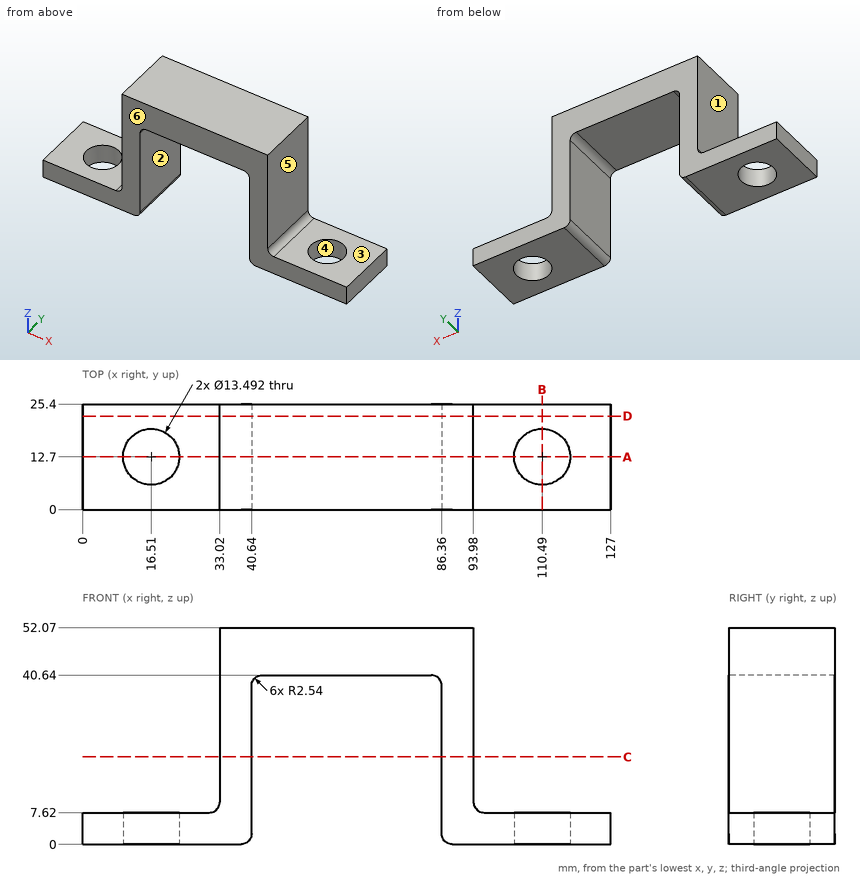
Answer from the drawing. Dimensions are ordinates in mm from the lowest x, y and z of the part. A direction names the side the tool comes from. Coordinates: 2 decimals unless noted, no trailing zeros. Write each loop counter-clockwise with the first axis right and the second up, starting at its lowest first coordinate (ties: lowest second). Pieces come first, ordered by that corner, then holes. Notation, with made-up numbers: (-1.75, 29) - (21.25, 29) arc R16 ccw to (21.25, 50) - close; hole circle Ø5 at (0, 77.5). An arc over 180 degrees is marked (long way). Return JSON: item names as keys, results as strings. Group by question number.
Q1. The part is cut by section B-B on x = 110.49. Write down the section's boundary in (y, z).
Q2. For a pull along X with two mould halves and no side action, classify the marked faces 4, 5 and 6 as +X half, -X half, draft (parallel to the pull), parting line (faces both ways), or undercut.
Q3. Which of the six approach directions +Z, -Z, +X, -X, +Y, -Y give full straight-line access (tool end or side, diameter ignored) to the marked faces 1, 2 and 3?
Q4. The part is cut by section A-A on y = 12.7. Write down the section's boundary in (x, z).
Q5. Find the intervals of material crossed by line 1 along X through (y, z) = (10.75, 25); line 2 along X through (y, z) = (11, 4.5); line 3 along Z through (x, y) = (97, 7), in increasing order. Write a range as [from, to].
Q6. The part is cut by section C-C on z = 21. Write down the section's boundary in (x, y), and give its area (3 significant figures).
Q7. The part is cut by section D-D on y = 22.5. Write down the section's boundary in (x, z), and give its area (3 significant figures).
Q8. Flat-ended cylindrical pins translate along their axes: pin 1 Ø7.5 at (x, y) = (60.5, 10.5) entering from -Z; pin 2 Ø12.5 at (y, z) = (15, 17) entering from -X; pin 3 Ø12.5 at (x, y) = (8, 10.5) entering from +Z. Find the tip coordinate at first contact, or state that the pin passes through.
Evaluation:
{
 "1": {"outline": "(0, 0) - (5.95, 0) - (5.95, 7.62) - (0, 7.62) - close; (19.45, 0) - (25.4, 0) - (25.4, 7.62) - (19.45, 7.62) - close"},
 "2": {"face 4": "undercut", "face 5": "+X half", "face 6": "draft"},
 "3": {"face 1": "+Z, -X, +Y, -Y", "face 2": "-Z, +Y, -Y", "face 3": "+Z, +X, +Y, -Y"},
 "4": {"outline": "(0, 0) - (9.76, 0) - (9.76, 7.62) - (0, 7.62) - close; (23.26, 0) - (38.1, 0) arc R2.54 ccw to (40.64, 2.54) - (40.64, 38.1) arc R2.54 cw to (43.18, 40.64) - (83.82, 40.64) arc R2.54 cw to (86.36, 38.1) - (86.36, 2.54) arc R2.54 ccw to (88.9, 0) - (103.74, 0) - (103.74, 7.62) - (96.52, 7.62) arc R2.54 cw to (93.98, 10.16) - (93.98, 52.07) - (33.02, 52.07) - (33.02, 10.16) arc R2.54 cw to (30.48, 7.62) - (23.26, 7.62) - close; (117.24, 0) - (127, 0) - (127, 7.62) - (117.24, 7.62) - close"},
 "5": {"line 1": "x = [33.02, 40.64], [86.36, 93.98]", "line 2": "x = [0, 9.98], [23.04, 40.64], [86.36, 103.96], [117.02, 127]", "line 3": "z = [0, 7.62]"},
 "6": {"outline": "(33.02, 0) - (40.64, 0) - (40.64, 25.4) - (33.02, 25.4) - close; (86.36, 0) - (93.98, 0) - (93.98, 25.4) - (86.36, 25.4) - close", "area": "387 mm2"},
 "7": {"outline": "(0, 0) - (38.1, 0) arc R2.54 ccw to (40.64, 2.54) - (40.64, 38.1) arc R2.54 cw to (43.18, 40.64) - (83.82, 40.64) arc R2.54 cw to (86.36, 38.1) - (86.36, 2.54) arc R2.54 ccw to (88.9, 0) - (127, 0) - (127, 7.62) - (96.52, 7.62) arc R2.54 cw to (93.98, 10.16) - (93.98, 52.07) - (33.02, 52.07) - (33.02, 10.16) arc R2.54 cw to (30.48, 7.62) - (0, 7.62) - close", "area": "1,820 mm2"},
 "8": {"pin 1": "stops at z = 40.64", "pin 2": "stops at x = 33.02", "pin 3": "stops at z = 7.62"}
}
